Verification items for the finished model (mm, model axes). Face numbers are marked on the shaded views. A direction names the side the tool comes from. Give positions to 0.01 mm unless a question says otherwise; leave off trailing zeros. Order: outer loops, then holes, each group sorted by start corner. A loop starts at its lowest first (then second) coordinate and runs counter-clockwise, first axis right, second up. Notation, with made-up numbers: (-28, 61.25) -> (-5, 61.25) arc R36 ccw to (-5, 98.25) -> close; hole circle Ø8 at (65, 9). An arc over 180 degrees is marked (long way). One line per question, with ' | ' between items. Start each with the question number.
Q1. Section check C-C on y = 8.75. Record the cut outline in (x, z).
Q2. Material ranges on probe 1 along X at (y, z) = (9.75, 5.5); probe 2 along Z at (x, y) = (59.5, 16); probe 3 along Y at (x, z) = (29.5, 8.5), recorded low to high. Write a range as [from, to].
Q3. Section check D-D on z = 27. Record the cut outline in (x, y).
Q4. Section check B-B on x = 48. Record the cut outline in (y, z), plus the area to 3 significant figures.
Q5. Access from +Z, -Z, +X, -X, +Y, -Y to the whole of each face (thin tool, end or side, straight path). Record for the marked faces 4, 5 and 6.
Q6. Go/stop test with flat-tipped pins: pin 1 (5 mm diameter, centred on x = 29, y = 16.5, fed in from +Z); pin 2 (1.5 mm diameter, centred on y = 3.5, z = 11, fed in from +X); pin 3 (8 mm diameter, centred on y = 6, z = 12.5, fed in from +X); pin 4 (6 mm diameter, centred on x = -1, z = 27, fed in from +Y). Record where each tip stops, or that it passes through.
Q7. Section check A-A on z = 8. Record the cut outline in (x, y).
Q8. Mould release check, pull along Y, two halves, no side actions. Record for the marked faces 1, 2 and 3: released by +Y, released by -Y, zero draft, split by the parting line, or undercut.
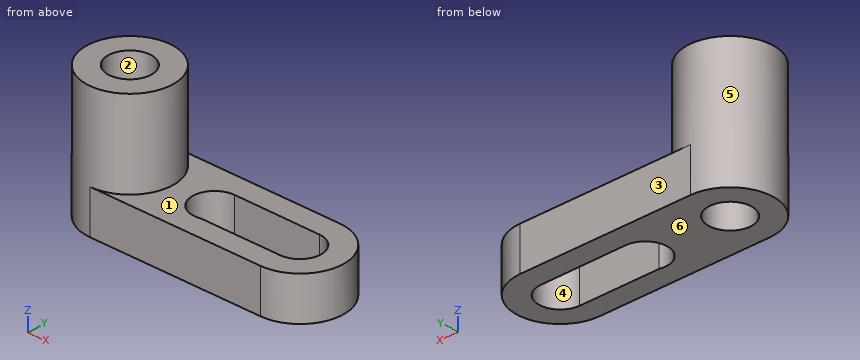
from build123d import *

# Parameters (mm, degrees)
F0_R     = 6.35
F1_DEPTH = 38.1
F3_DEPTH = 25.4


with BuildPart() as f1:
    # F0 (on Top) → F1 (new body)
    with BuildSketch(Plane.XY):
        with BuildLine():
            ThreePointArc((0, 25.4), (-12.7, 12.7), (0, 0))
            Line((0, 0), (50.8, 0))
            ThreePointArc((50.8, 0), (63.535209, 12.682377), (50.835197, 25.4))
            Line((50.835197, 25.4), (0, 25.4))
        make_face()
        with BuildLine():
            Line((25.483008, 18.937421), (50.88276, 18.825148))
            ThreePointArc((50.88276, 18.825148), (57.072841, 12.563859), (50.835197, 6.349951))
            Line((50.835197, 6.349951), (27.129976, 6.349951))
            ThreePointArc((27.129976, 6.349951), (19.103581, 11.701243), (25.483008, 18.937421))
        make_face(mode=Mode.SUBTRACT)
        with Locations((0, 12.7)):
            Circle(F0_R, mode=Mode.SUBTRACT)
    extrude(amount=F1_DEPTH)

    # F2 (on face) → F3 (cut)
    with BuildSketch(Plane.XY.offset(38.1)):
        with BuildLine():
            ThreePointArc((0, 25.4), (12.7, 12.7), (0, 0))
            Line((0, 0), (50.8, 0))
            ThreePointArc((50.8, 0), (63.535209, 12.682377), (50.835197, 25.4))
            Line((50.835197, 25.4), (0, 25.4))
        make_face()
        with BuildLine():
            Line((50.835197, 6.349951), (27.129976, 6.349951))
            ThreePointArc((27.129976, 6.349951), (19.103581, 11.701243), (25.483008, 18.937421))
            Line((25.483008, 18.937421), (50.88276, 18.825148))
            ThreePointArc((50.88276, 18.825148), (57.072841, 12.563859), (50.835197, 6.349951))
        make_face(mode=Mode.SUBTRACT)
    extrude(amount=-F3_DEPTH, mode=Mode.SUBTRACT)


solid = f1.part
Filled in:
1) outline: (-12.07, 0) -> (-4.97, 0) -> (-4.97, 38.1) -> (-12.07, 38.1) -> close; (4.97, 0) -> (20.29, 0) -> (20.29, 12.7) -> (12.07, 12.7) -> (12.07, 38.1) -> (4.97, 38.1) -> close; (55.75, 0) -> (62.91, 0) -> (62.91, 12.7) -> (55.75, 12.7) -> close
2) probe 1: [-12.35, -5.62], [5.62, 19.69], [56.39, 63.19] | probe 2: [0, 12.7] | probe 3: [0, 6.35], [18.92, 25.4]
3) outline: circle Ø25.4 at (0, 12.7); hole circle Ø12.7 at (0, 12.7)
4) outline: (0, 0) -> (6.35, 0) -> (6.35, 12.7) -> (0, 12.7) -> close; (18.84, 0) -> (25.4, 0) -> (25.4, 12.7) -> (18.84, 12.7) -> close | area: 164 mm²
5) face 4: +Z, -Z | face 5: +Z | face 6: -Z, +X, -X, +Y, -Y
6) pin 1: z = 12.7 | pin 2: x = 60.32 | pin 3: x = 63.24 | pin 4: y = 25.4
7) outline: (0, 0) -> (50.8, 0) arc R12.7 ccw to (50.84, 25.4) -> (0, 25.4) arc R12.7 ccw to start; hole circle Ø12.7 at (0, 12.7); hole (25.48, 18.94) arc R6.41 ccw (long way) to (27.13, 6.35) -> (50.84, 6.35) arc R6.24 ccw to (50.88, 18.83) -> close
8) face 1: zero draft | face 2: undercut | face 3: released by +Y
